Design review of the part built by this model. Coordinates are the model's own, in mm. A direction names the side the tool comes from. Coordinates: 2 decimals unless noted, no trailing zeros. Write each loop counter-clockwise with the first axis right and the second up, starting at its lowest first coordinate (ties: lowest second). Pieces come first, ordered by that corner, then holes.
```python
from build123d import *

# Parameters (mm, degrees)
F0_W     = 6.35
F0_H     = 12.7
F1_DEPTH = 19.05
F2_W     = 6.35
F2_H     = 12.7
F3_DEPTH = 6.35
F4_W     = 12.7
F4_H     = 6.35
F5_DEPTH = 6.35


with BuildPart() as f1:
    # F0 (on Right) → F1 (new body)
    with BuildSketch(Plane.YZ):
        Polygon((-27.807808, 12.414332), (-21.457808, 12.414332), (-21.457808, 25.114332), (-8.757808, 25.114332), (-8.757808, 31.464332), (-21.457808, 31.464332), (-27.807808, 31.464332), (-40.507808, 31.464332), (-40.507808, 25.114332), (-27.807808, 25.114332), align=None)
        with Locations((-24.632808, 37.814332)):
            Rectangle(F0_W, F0_H)
    extrude(amount=F1_DEPTH)

    # F2 (on face) → F3 (join)
    with BuildSketch(Plane.YZ.offset(19.05)):
        with Locations((-24.632808, 37.814332)):
            Rectangle(F2_W, F2_H)
    extrude(amount=F3_DEPTH)

    # F4 (on face) → F5 (cut)
    with BuildSketch(Plane.YZ.offset(19.05)):
        with Locations((-34.157808, 28.289332)):
            Rectangle(F4_W, F4_H)
    extrude(amount=-F5_DEPTH, mode=Mode.SUBTRACT)


solid = f1.part
```
(1) For faces 4 (the flat face through (9, -21.458, 19)), 5 (the flat face through (6, -34, 25.114)), 6 (the flat face through (9, -15, 31.464)), list the 3-axis set-ups (+Z, -Z, +X, -X, +Y, -Y) from which the entire face can be reached by the end or side of a thin tool; tool diameter is ignored.
(2) Consider section A-A (x = 4.5). Give the boundary of the cut face in (y, z).
(3) Mouldability with a two-part tool opening along Z and no side actions: class faces 1 (the flat face through (6, -34, 31.464)), 2 (the flat face through (9, -15, 25.114)), 3 (the flat face through (13, -27.808, 32)) as +Z half, -Z half, draft (parallel to the pull), parting line (faces both ways), or undercut.
(4) Wall thickness on line 1 (Z direction, x = 6, y = -34.5); line 2 (Y direction, x = 13.5, z = 41); line 3 (X direction, y = -14, z = 30.5): over which ranges is each line inside the solid? List them lowest first.
(5) Consider section C-C (z = 29). Give the boundary of the cut face in (x, y).
(6) Insertion check: pin 1 Ø4 at (x, y) = (13.5, -16.5) entering from +Z; pin 2 Ø14 at (x, z) = (12, 39.5) entering from +Y; pin 3 Ø7 at (y, z) = (-32, 29.5) entering from +X. Each pin has a flat end and moves straight along its axis. Give the tip position at first contact, or say it passes through.
(7) Consider section D-D (y = -30). Give the boundary of the cut face in (x, z), plus the area to 3 significant figures.
(8) Consider section B-B (y = -20). Give the boundary of the cut face in (x, z), plus the area to 3 significant figures.
Results:
1. face 4: -Z, +X, -X, +Y
1. face 5: -Z, +X, -X, -Y
1. face 6: +Z, +X, -X, +Y
2. outline: (-40.51, 25.11) - (-27.81, 25.11) - (-27.81, 12.41) - (-21.46, 12.41) - (-21.46, 25.11) - (-8.76, 25.11) - (-8.76, 31.46) - (-21.46, 31.46) - (-21.46, 44.16) - (-27.81, 44.16) - (-27.81, 31.46) - (-40.51, 31.46) - close
3. face 1: +Z half
3. face 2: -Z half
3. face 3: draft
4. line 1: z = 25.11 to 31.46
4. line 2: y = -27.81 to -21.46
4. line 3: x = 0 to 19.05
5. outline: (0, -40.51) - (12.7, -40.51) - (12.7, -27.81) - (19.05, -27.81) - (19.05, -8.76) - (0, -8.76) - close
6. pin 1: stops at z = 31.46
6. pin 2: stops at y = -21.46
6. pin 3: stops at x = 12.7
7. outline: (0, 25.11) - (12.7, 25.11) - (12.7, 31.46) - (0, 31.46) - close
7. area: 80.6 mm2
8. outline: (0, 25.11) - (19.05, 25.11) - (19.05, 31.46) - (0, 31.46) - close
8. area: 121 mm2
